Part print with two shaded views. Sizes in mm from the minimum x, y, z corner. A direction names the side the tool comes from. Coordinates: 2 decimals unless noted, no trailing zeros. Loops run counter-clockwise (first coordinate to the right, second up) from the corner with the lowest first, then second, coordinate; pieces in that order, holes last.
Item 1: Cut at B-B (y = 28.5). List the corners of the cut face in (x, z) (1 decimal).
Item 2: Flat gauge pins, fed straight in: pin 1 (1.3 mm diameter, centred on x = 1.5, y = 13, fed in from +Z); pin 2 (4 mm diameter, centred on x = 104.5, z = 34.5, fed in from +Y); pin 3 (12 mm diameter, centred on x = 87, z = 36, fed in from +Y). Where does each tip first touch, or does it go through?
Item 3: Drill centre lines: line 1 along X through (y, z) = (24, 38.5) (1 decimal); line 2 along Y through (x, z) = (98.5, 14.5); line 3 along Y through (x, z) = (42.5, 46) (1 decimal). Where is each one in solid material? Low to high.
Item 4: Cut at A-A (x = 90). List the corners of the cut face in (y, z).
Item 5: Mould opens along Y. For the marked faces 1, 2, 3 and 4 say: released by +Y, released by -Y, zero draft, split by the parting line, or undercut.
Item 6: Cut at C-C (z = 36). List the corners of the cut face in (x, y) (1 decimal).
Item 7: 3-axis set-ups, long thin cutter, end or side, ignore diameter. For the marked faces 5, 6 and 7: which of +Z, -Z, +X, -X, +Y, -Y reach the whole face in a straight line?
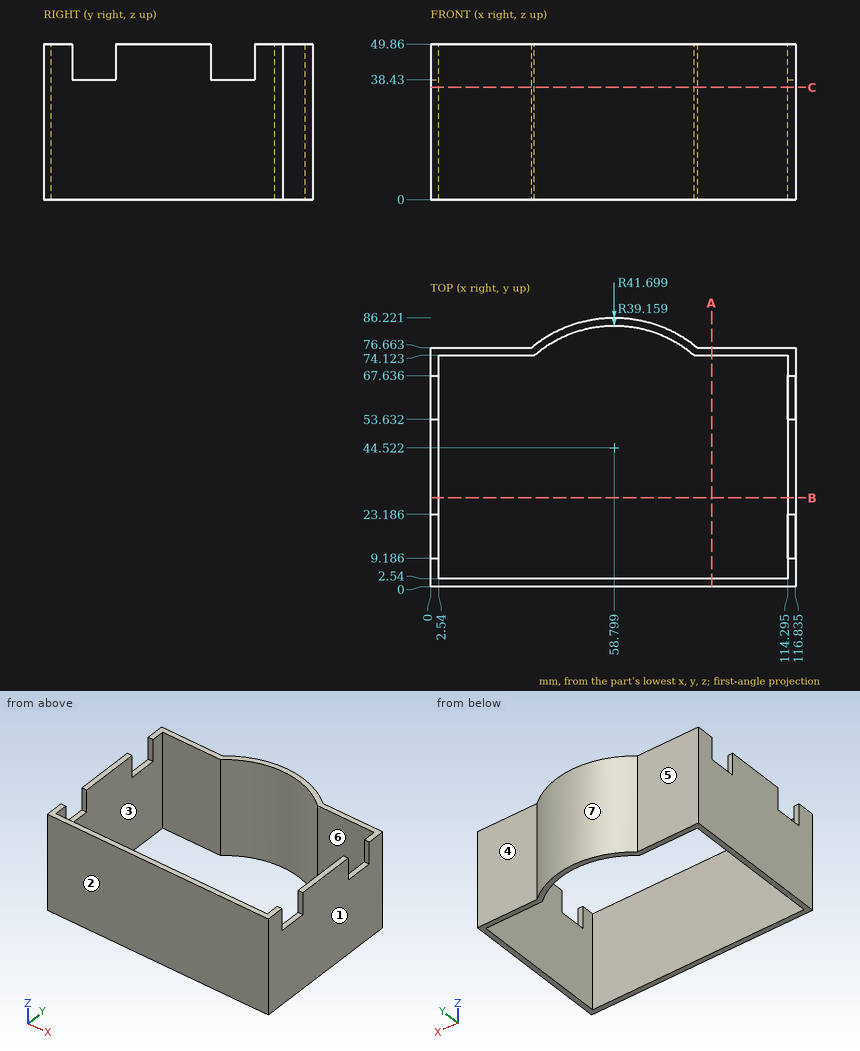
Filled sheet:
1. outline: (0, 0) - (2.5, 0) - (2.5, 49.9) - (0, 49.9) - close; (114.3, 0) - (116.8, 0) - (116.8, 49.9) - (114.3, 49.9) - close
2. pin 1: stops at z = 38.43
2. pin 2: stops at y = 76.66
2. pin 3: stops at y = 79.82
3. line 1: x = 0 to 2.5, 114.3 to 116.8
3. line 2: y = 0 to 2.54, 74.12 to 76.66
3. line 3: y = 0 to 2.5, 80.1 to 82.9
4. outline: (0, 0) - (2.54, 0) - (2.54, 49.86) - (0, 49.86) - close; (74.12, 0) - (76.66, 0) - (76.66, 49.86) - (74.12, 49.86) - close
5. face 1: zero draft
5. face 2: released by -Y
5. face 3: undercut
5. face 4: released by +Y
6. outline: (0, 0) - (116.8, 0) - (116.8, 76.7) - (85.4, 76.7) arc R41.7 ccw to (32.2, 76.7) - (0, 76.7) - close; hole (2.5, 2.5) - (114.3, 2.5) - (114.3, 74.1) - (84.4, 74.1) arc R39.2 ccw to (33.2, 74.1) - (2.5, 74.1) - close
7. face 5: +Z, -Z, -X, +Y
7. face 6: +Z, -Z
7. face 7: +Z, -Z, +Y
